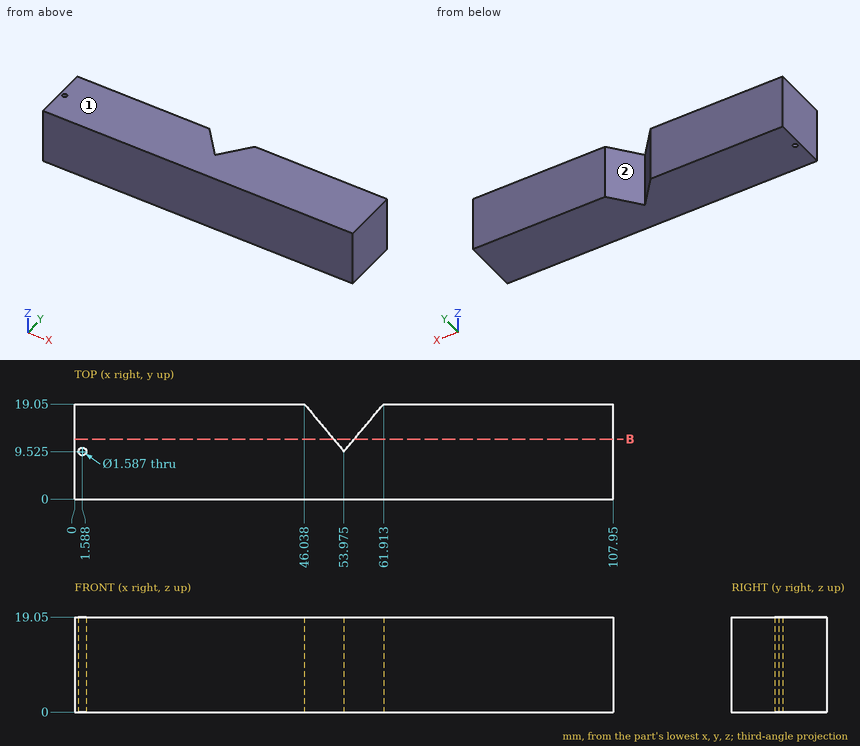
Can you work these out from the drawing? Everything is in mm from the part's minimum corner. A direction names the side the tool comes from. Round coordinates to 2 decimals unless told otherwise and drop trailing zeros. Loops run counter-clockwise (first coordinate to the right, second up) from the corner with the lowest first, then second, coordinate; pieces in that order, holes last.
1. Which directions (+Z, -Z, +X, -X, +Y, -Y) give clear straight access to the entire face, cutting with the end or side of a thin tool? Please do the marked faces 1 and 2.
Answer list:
face 1: +Z, +X, -X, +Y, -Y
face 2: +Z, -Z, +Y
2. If we section it at B-B on y = 12: Write out the boundary of the cut face in (x, z), plus the area to 3 significant figures.
Answer list:
outline: (0, 0) - (51.91, 0) - (51.91, 19.05) - (0, 19.05) - close; (56.04, 0) - (107.95, 0) - (107.95, 19.05) - (56.04, 19.05) - close
area: 1,980 mm2
3. If I drill on line 1 along X through (y, z) = (17.5, 6.25); line 2 along X through (y, z) = (11.5, 11.75); line 3 along Y through (x, z) = (55.5, 9.75) (1 decimal), over which ranges is the centre line in solid material (lowest first)?
Answer list:
line 1: x = 0 to 47.33, 60.62 to 107.95
line 2: x = 0 to 52.33, 55.62 to 107.95
line 3: y = 0 to 11.4
4. For P1, Ø1, axis at x = 1.59, y = 9.52, coming from the -Z side, with a flat end and sliding along its axis, tell me the tip position at first contact or that it passes through.
Answer list:
P1: passes through
